For this review, use the dimensioned drawing (mm, ordinates from the lowest corner) and the shaded views. A direction names the side the tool comes from. Round coordinates to 2 decimals unless told otherwise and drop trailing zeros. Order: outer loops, then holes, each group sorted by start corner. A loop starts at its lowest first (then second) coordinate and runs counter-clockwise, first axis right, second up. Notation, with made-up numbers: M 31,-24 L 87,-24 A29 ccw 87,15 Z; hole C -2,72 d9. An arc over 180 degrees is marked long. One line per item, written item: value. Start each with the question number.
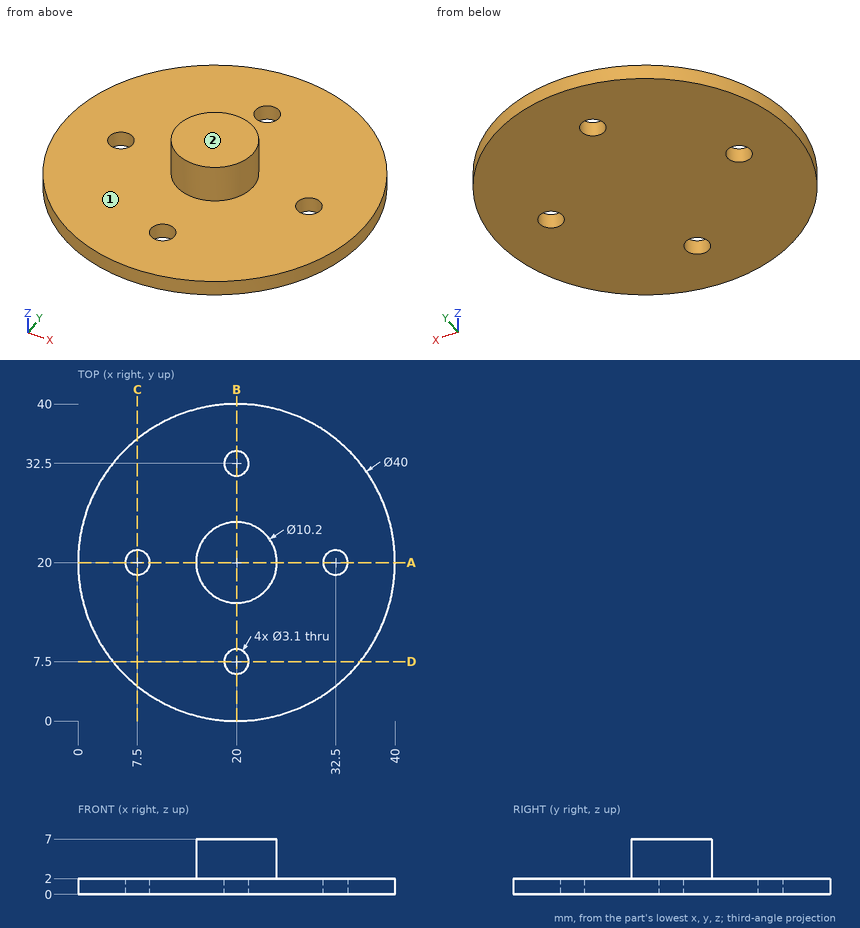
Item 1: Consider section C-C, the plane x = 7.5. Give the boundary of the cut face in (y, z).
Item 2: Consider section A-A, the plane y = 20. Give the boundary of the cut face in (x, z).
Item 3: Clearance check with flat-ended pins moving along their axes: P1, Ø3, axis at x = 19, z = 1.5, coming from the -Y side; P2, Ø1, axis at y = 21.5, z = 5, coming from the -X side; P3, Ø8, axis at x = 30.5, y = 4.5, coming from the +Z side. State where each tip first meets the part, or that it passes through.
Item 4: Machinability: for the marked faces 1 and 2, which of the approach directions +Z, -Z, +X, -X, +Y, -Y give a long, thin tool a straight path to every point of the face, cutting with its end or side? Answer none if there is none.
Item 5: Wall thickness on L1, parallel to Z at x = 26.5, y = 19; L2, parallel to X at y = 21, z = 0.75; L3, parallel to Y at x = 7, z = 1.5: over which ranges is each line inside the solid? List them lowest first.
Computed:
1. outline: M 4.39,0 L 18.45,0 L 18.45,2 L 4.39,2 Z; M 21.55,0 L 35.61,0 L 35.61,2 L 21.55,2 Z
2. outline: M 0,0 L 5.95,0 L 5.95,2 L 0,2 Z; M 9.05,0 L 30.95,0 L 30.95,2 L 25.1,2 L 25.1,7 L 14.9,7 L 14.9,2 L 9.05,2 Z; M 34.05,0 L 40,0 L 40,2 L 34.05,2 Z
3. P1: stops at y = 0
3. P2: stops at x = 15
3. P3: stops at z = 2
4. face 1: +Z
4. face 2: +Z, +X, -X, +Y, -Y
5. L1: z = 0 to 2
5. L2: x = 0.03 to 6.32, 8.68 to 31.32, 33.68 to 39.97
5. L3: y = 4.8 to 18.53, 21.47 to 35.2
